Geometry check sheet. Reference: the model listing, model coordinates, mm. A direction names the side the tool comes from. Coordinates: 2 decimals unless noted, no trailing zeros. Loops run counter-clockwise (first coordinate to the right, second up) from the corner with the lowest first, then second, coordinate; pieces in that order, holes last. Notation, with made-up numbers: (53, -19.75) -> (86, -19.75) arc R5 ccw to (86, -12.75) -> close; hole circle Ø9 at (-6, -1). An arc over 180 degrees is marked (long way). Answer as a JSON object with one key per item and string values.
from build123d import *


with BuildPart() as part:
    # Эскиз1 → Повернуть1 (revolve)
    with BuildSketch(Plane.XY):
        with BuildLine():
            Line((11.5, -2.982243983), (11.5, -5.627433044))
            Line((11.5, -5.627433044), (6, -5.627433044))
            Line((6, -5.627433044), (6, 2.372566956))
            Line((6, 2.372566956), (0, 3.372566956))
            Line((0, 3.372566956), (0, 4.372566956))
            ThreePointArc((0, 4.372566956), (4.029595345, 4.302809639), (8, 3.611151047))
            Line((8, 3.611151047), (8, 3.372566956))
            Line((8, 3.372566956), (7, 3.372566956))
            Line((7, 3.372566956), (7, 2.372566956))
            Line((7, 2.372566956), (11.5, 2.372566956))
            Line((11.5, 2.372566956), (11.5, -0.481527002))
            Line((11.5, -0.481527002), (10, -0.470528934))
            Line((10, -0.470528934), (10, -2.971245915))
            Line((10, -2.971245915), (11.5, -2.982243983))
        make_face()
    revolve(axis=Axis((0, 3.372566956, 0), (0, 1, 0)))


solid = part.part
1. Section check A-A, the plane y = -1. Record the boundary of the cut face in (x, z), then the cut area to 3 significant figures.
Evaluation:
{"outline": "circle Ø20 at (0, 0); hole circle Ø12 at (0, 0)", "area": "201 mm^2"}
2. Thickness scan on probe 1 along Y at (x, z) = (10.75, -1.5); probe 2 along Z at (x, y) = (0, 0); probe 3 along Z at (x, y) = (0, -2.25). Record the ranges inside material, lowest first. Write a range as from..to.
Evaluation:
{"probe 1": "y = -5.63..-2.98, -0.48..2.37", "probe 2": "z = -11.5..-6, 6..11.5", "probe 3": "z = -10..-6, 6..10"}
3. Depth check by flat-ended pin: P1, Ø5, axis at x = 2, z = 1, coming from the -Y side; P2, Ø1.5, axis at y = 0, z = -6.5, coming from the -X side; P3, Ø10, axis at x = -0.5, z = 7, coming from the +Y side. Enter the tip coordinate at first touch or a pass-through.
Evaluation:
{"P1": "stops at y = 2.58", "P2": "stops at x = -9.96", "P3": "stops at y = 4.42"}
4. Mould release check, pull along Y, two halves, no side actions. Record for faces 3 (the face through (0, 2.373, 8)), 4 (the face through (-6, -2, 0)), 5 (the face through (5, -5.627, 5)): released by +Y, released by -Y, zero draft, split by the parting line, or undercut.
Evaluation:
{"face 3": "undercut", "face 4": "zero draft", "face 5": "released by -Y"}
5. Tool access check on faces 1 (the face through (6.466, 2.866, 2.681)), 2 (the face through (-0.063, 3.324, 0.284)). Record the directions out of +Z, -Z, +X, -X, +Y, -Y that give a thin tool (end or side, any length) a straight path to the whole face; none if there is none.
Evaluation:
{"face 1": "none", "face 2": "-Y"}
